Autodesk Fusion 360 part; units mm, degrees
sketch "Sketch1" plane through (0, 0, 0) normal (0, 1, 0) x (1, 0, 0)
  line L0 (-0.5, 0) -> (0.5, 0)
  line L1 (-0.2, 0) -> (-0.2, -0.6)
  line L2 (-0.2, -0.6) -> (-1, -1.9856)
  line L3 (-1, -1.9856) -> (-1, -12.0716)
  line L4 (-4.4259, -12.5) -> (0, -12.5)
  line L5 (0, -12.5) -> (0, 0)
  line L6 (-1, -12.0716) -> (-1.3, -12.5)
  line L7 (-1.3, -12.5) -> (-4.4259, -12.5)
  line L8 (-0.5, 0) -> (-1.8407, -1.9147)
  arc A0 (-0.3959, 0) -> (-0.5597, -0.0853) centre (-0.3959, -0.2) ccw
  line L9 (-2.0045, -2) -> (-3.5, -2)
  line L10 (-3.5, -2) -> (-3.5, -5)
  line L11 (-3.5, -5) -> (-2.7, -5)
  line L12 (-2.5, -5.2) -> (-2.5, -6)
  line L13 (-2.5, -6) -> (-3, -6.5)
  line L14 (-3, -6.5) -> (-3, -12)
  line L15 (-3, -12) -> (-2.5, -12.5)
  arc A1 (-2.0045, -2) -> (-1.8407, -1.9147) centre (-2.0045, -1.8) ccw
  arc A2 (-2.5, -5.2) -> (-2.7, -5) centre (-2.7, -5.2) ccw
  point P0 (-1.9004, -2)
  dimension "d3" = 0.2
  dimension "d5" = 30
  dimension "d10" = 12.5
  dimension "d11" = 1.3
  dimension "d12" = 1
  dimension "d14" = 125
  dimension "d15" = 0.6
  dimension "d16" = 1
  dimension "d17" = 0.2
  dimension "d18" = 2
  dimension "d19" = 3.5
  dimension "d20" = 5
  dimension "d21" = 2.5
  dimension "d24" = 3
  dimension "d25" = 135
  dimension "d26" = 135
  dimension "d27" = 0.5
  dimension "d28" = 1
  dimension "d29" = 0.2
  dimension "d38" = 0.2
revolve "Revolve1" add sketch "Sketch1" angle 360 about axis through (0, 0, 12.5) along (0, 0, -1) contours L0 L1 L2 L3 L4 L6 L7 L8 A0 L9 L10 L11 L12 L13 L14 L15 A1 A2
sketch "Sketch2" plane through (0, 0, 2) normal (0, 0, -1) x (1, 0, 0)
  circle A0 centre (0, 0) radius 3.5
  circle A1 centre (0, 0) radius 2.0045
  line L0 (-3.5, -2.0207) -> (0, -4.0415)
  line L1 (0, -4.0415) -> (3.5, -2.0207)
  line L2 (3.5, -2.0207) -> (3.5, 2.0207)
  line L3 (3.5, 2.0207) -> (0, 4.0415)
  line L4 (0, 4.0415) -> (-3.5, 2.0207)
  line L5 (-3.5, 2.0207) -> (-3.5, -2.0207)
  line L6 (-0.1584, 3.95) -> (0.1584, 3.95)
  line L7 (-0.1584, -3.95) -> (0.1584, -3.95)
  line L8 (0, 3.95) -> (0, -3.95) construction
  line L9 (-3.3416, -2.1122) -> (-3.5, -1.8378)
  line L10 (3.5, 1.8378) -> (3.3416, 2.1122)
  line L11 (3.5, -1.8378) -> (3.3416, -2.1122)
  line L12 (-3.3416, 2.1122) -> (-3.5, 1.8378)
  dimension "d31" = 7.9
  dimension "d33" = 360
extrude "Extrude1" add sketch "Sketch2" against normal up to surface (3 mm away) contours A0 L1 L2 L11 | A0 L2 L3 L10 | A0 L3 L4 L6 | A0 L0 L1 L7 | A0 L4 L5 L12 | A0 L0 L5 L9
fillet "Fillet1" radius 0.2 12 edges at (3.4208, -1.975, 2) (3.4208, -1.975, 5) (0, -3.95, 5) (0, -3.95, 2) (-3.4208, -1.975, 2) (-3.4208, -1.975, 5) (-3.4208, 1.975, 5) (-3.4208, 1.975, 2) (0, 3.95, 5) (0, 3.95, 2) (3.4208, 1.975, 2) (3.4208, 1.975, 5)
equation "Table_D = 2 mm"
equation "d3 = Nozzle_Diameter / 2"
equation "Nozzle_Diameter = 0.4 mm"
equation "Table_C = 0.6 mm"
equation "Table_B = 1 mm"
equation "Table_F = 0.2 mm"
equation "Table_E = 2.6 mm"
equation "d11 = Table_E / 2"
equation "d12 = Table_D / 2"
equation "d15 = Table_C"
equation "d16 = Table_B"
equation "d17 = Table_F"
equation "d26 = d25"
equation "d29 = Table_F"
equation "d37 = Table_F"
Input: part model. Units: mm. Frame: model coordinates. A direction names the side the tool comes from. Give positions to 0.01 mm unless a question says otherwise; leave off trailing zeros. Loops run counter-clockwise (first coordinate to the right, second up) from the corner with the lowest first, then second, coordinate; pieces in that order, holes last. Notation, with made-up numbers: M 45.5,44.25 L 74.5,44.25 A32 cw 74.5,74.25 Z; hole C 13.25,46 d1. An arc over 180 degrees is marked long. Use CSV: the item, a comma, the result in double quotes.
(1) Pull-direction query (Z, two-part tool) for faces 4 (the face through (-3.5, 0, 3)), 5 (the face through (2, 2, 2)), 6 (the face through (0.54, 2.44, 5.61)); classes: pulls with the +Z half, pulls with the -Z half, needs draft (parallel to the pull), parting line crosses it, or undercut.
Outcome:
face 4,"needs draft"
face 5,"pulls with the -Z half"
face 6,"undercut"
(2) Section B-B, the plane z = 8.5. Return loops of the section in (x, y), plus the area to 3 significant figures.
Outcome:
outline,"C 0,0 d6; hole C 0,0 d2"
area,"25.1 mm²"
(3) Set-up query: faces 1 (the face through (-1.728, -3.044, 3.479)), 2 (the face through (3, 0, 9)), 3 (the face through (3, 1, 5)). Return all of +Z, -Z, +X, -X, +Y, -Y with unobstructed straight access to the full face (end or side cutting, diameter ignored); none if empty.
Outcome:
face 1,"+Z, -Z, -X, -Y"
face 2,"+Z"
face 3,"none"
(4) Pin query (flat end, axial travel): P1, Ø1, axis at y = 1, z = 6.5, coming from the +X side; P2, Ø2, axis at x = 3, y = -3, coming from the -Z side. Return the tip coordinate at first contact, or that it passes through.
Outcome:
P1,"stops at x = 2.96"
P2,"stops at z = 2"
(5) Material intervals for L1, parallel to Y at x = 0, z = 8.5; L2, parallel to Z at x = 0.5, y = -2.5; L3, parallel to Z at x = 2, y = -1, sorted ascending. Write a range as [from, to].
Outcome:
L1,"y = [-3, -1], [1, 3]"
L2,"z = [2, 5.07], [6.05, 12.45]"
L3,"z = [2, 12.5]"
(6) Section C-C, the plane z = 3. Return loops of the section in (x, y).
Outcome:
outline,"M -3.5,-1.84 L -3.34,-2.11 L -0.16,-3.95 L 0.16,-3.95 L 3.34,-2.11 L 3.5,-1.84 L 3.5,1.84 L 3.34,2.11 L 0.16,3.95 L -0.16,3.95 L -3.34,2.11 L -3.5,1.84 Z; hole C 0,0 d2"
